For this review, take the finished solid that the model builds, in its own axes (mm). A direction names the side the tool comes from. Round coordinates to 2 decimals unless told otherwise and drop trailing zeros. Loops run counter-clockwise (first coordinate to the right, second up) from the corner with the lowest first, then second, coordinate; pieces in that order, holes last. Notation, with made-up numbers: (69, 15.25) -> (85, 15.25) arc R31 ccw to (85, 39.25) -> close; hole circle Ø9 at (-0.5, 48). An arc over 180 degrees is marked (long way). Use one line per item in the form item = value. Start each with the question number.
from build123d import *

# Parameters (mm, degrees)
F0_R      = 14.25
F1_DEPTH  = 1
F2_R      = 7.430853
F3_DEPTH  = 10.3
F4_R      = 14.25
F5_DEPTH  = 20.3
F6_R      = 5
F7_R      = 1.5
F8_DEPTH  = 16.7
F9_R      = 1.5
F10_DEPTH = 1


with BuildPart() as f1:
    # F0 (on Top) → F1 (new body)
    with BuildSketch(Plane.XY):
        Circle(F0_R)
    extrude(amount=F1_DEPTH)

    # F2 (on face) → F3 (join)
    with BuildSketch(Plane.XY.offset(1)):
        Circle(F2_R)
    extrude(amount=F3_DEPTH)

    # F4 (on face) → F5 (join)
    with BuildSketch(Plane.XY.offset(11.3)):
        Circle(F4_R)
    extrude(amount=F5_DEPTH)

    # F6
    f6_edges = [f1.edges().sort_by_distance(p)[0] for p in [
        (-14.25, 0, 31.6),
    ]]
    fillet(f6_edges, radius=F6_R)

    # F7 (on face) → F8 (join)
    with BuildSketch(Plane.XY.offset(31.6)):
        Circle(F7_R)
    extrude(amount=F8_DEPTH)

    # F9 (on face) → F10 (cut, through all)
    with BuildSketch(Plane(origin=(0, 0, 0), x_dir=(1, 0, 0), z_dir=(0, 0, -1))):
        with Locations((0, 11)):
            Circle(F9_R)
        with Locations((11, 0)):
            Circle(F9_R)
        with Locations((-11, 0)):
            Circle(F9_R)
        with Locations((0, -11)):
            Circle(F9_R)
    extrude(amount=-F10_DEPTH, mode=Mode.SUBTRACT)


solid = f1.part
Item 1: Take a section at A-A on x = 0. Give the boundary of the cut face in (y, z), plus the area to 3 significant figures.
Item 2: Machinability: for faces 4 (the flat face through (0, 0, 48.3)), 5 (the cylindrical face through (-1.611, -7.254, 6.078)), 6 (the cylindrical face through (-12.5, -0.07, 0.49)), which of the approach directions +Z, -Z, +X, -X, +Y, -Y give a long, thin tool a straight path to every point of the face, cutting with its end or side? Answer none if there is none.
Item 3: Wall thickness on line 1 (Y direction, x = 0, z = 0.55); line 2 (Z direction, x = 4, y = -7.5); line 3 (Z direction, x = 7.75, y = -9): over which ranges is each line inside the solid? List them lowest first.
Item 4: Draft analysis for pull direction Z (two halves, no side actions). For faces 1 (the flat face through (6, -6, 1)), 2 (the cylindrical face through (-1.5, 0.07, 39.83)), 3 (the flat face through (2, 0, 31.6)), state which applies: +Z half, -Z half, draft (parallel to the pull), parting line (faces both ways), or undercut.
Item 5: For P1, Ø10, axis at x = 1, z = 37, coming from the -Y side; P2, Ø1.8, axis at x = 11, y = 0, coming from the -Z side; P3, Ø2, axis at x = -3, z = 25, coming from the -Y side, all flat-tipped, find the tip position at first contact; note any pin that passes through.
Item 6: Take a section at C-C on z = 9. Give the boundary of the cut face in (x, y).
Item 7: Take a section at D-D on z = 44. Give the boundary of the cut face in (x, y).
Results:
q1.outline = (-14.25, 0) -> (-12.5, 0) -> (-12.5, 1) -> (-14.25, 1) -> close; (-14.25, 11.3) -> (-7.43, 11.3) -> (-7.43, 1) -> (-9.5, 1) -> (-9.5, 0) -> (9.5, 0) -> (9.5, 1) -> (7.43, 1) -> (7.43, 11.3) -> (14.25, 11.3) -> (14.25, 26.6) arc R5 ccw to (9.25, 31.6) -> (1.5, 31.6) -> (1.5, 48.3) -> (-1.5, 48.3) -> (-1.5, 31.6) -> (-9.25, 31.6) arc R5 ccw to (-14.25, 26.6) -> close; (12.5, 0) -> (14.25, 0) -> (14.25, 1) -> (12.5, 1) -> close
q1.area = 793 mm2
q2.face_4 = +Z, +X, -X, +Y, -Y
q2.face_5 = none
q2.face_6 = -Z
q3.line_1 = -14.25 to -12.5, -9.5 to 9.5, 12.5 to 14.25
q3.line_2 = 0 to 1, 11.3 to 31.6
q3.line_3 = 0 to 1, 11.3 to 30.85
q4.face_1 = undercut
q4.face_2 = draft
q4.face_3 = +Z half
q5.P1 = -1.5
q5.P2 = 11.3
q5.P3 = -14.11
q6.outline = circle Ø14.86 at (0, 0)
q7.outline = circle Ø3 at (0, 0)
